Model file for the job. Use its own axes, mm. Face numbers are marked on the shaded views. A direction names the side the tool comes from. Give positions to 0.01 mm unless a question says otherwise; leave off trailing zeros. Order: outer loops, then holes, each group sorted by start corner. A loop starts at its lowest first (then second) coordinate and runs counter-clockwise, first axis right, second up. Notation, with made-up numbers: (53.25, 8) -> (79.25, 8) arc R22 ccw to (79.25, 40) -> close; hole circle Ø4 at (-27, -1.75). An arc over 180 degrees is marked (long way). Use CSV: the item, a comma, the result in double quotes. Start each with the question number.
1. Drop flat-ended pins along their axis: pin 1 (2 mm diameter, centred on x = 2.5, z = -27.5, fed in from +Y); pin 2 (2.5 mm diameter, centred on x = 1.5, y = -6.5, fed in from -Z); pin 3 (0.7 mm diameter, centred on x = 2, y = -9, fed in from -Z). Give the stop position or say it passes through.
2. Cut at D-D on z = -19. List the corners of the cut face in (x, y).
3. Cut at C-C on y = -13. List the corners of the cut face in (x, z), then the cut area to 3 significant figures.
4. Cut at A-A on x = 0.95. Give the number of separate pieces and of enclosed holes in the cut face, then the cut area to 3 significant figures.
5. Cut at B-B on z = -8. List the corners of the cut face in (x, y).
6. Wall check: line 1 (Z direction, x = 2.15, y = -14.5); line 2 (Y direction, x = 0.8, z = -1); line 3 (Y direction, x = 0.25, z = -3). Give the ranges that are in metal, low to high. Write a range as from..to.
7. 3-axis set-ups, long thin cutter, end or side, ignore diameter. For the marked faces 4, 5 and 6: which of +Z, -Z, +X, -X, +Y, -Y reach the whole face in a straight line?
8. Pull direction Y, two halves, no side cores. Call the marked faces 1, 2 and 3: released by +Y, released by -Y, zero draft, split by the parting line, or undercut.
```python
from build123d import *

# Parameters (mm, degrees)
F1_W     = 5
F1_H     = 5
F2_DEPTH = 5


with BuildPart() as f2:
    # F1 (on Right) → F2 (new body)
    with BuildSketch(Plane.YZ):
        with BuildLine():
            Line((-3.5, 0), (0, 0))
            Line((0, 0), (0, 8))
            ThreePointArc((0, 8), (-0.5857864376, 9.4142135624), (-2, 10))
            Line((-2, 10), (-20.8578643763, 10))
            ThreePointArc((-20.8578643763, 10), (-28.5115330236, 8.4775906502), (-35, 4.1421356237))
            Line((-35, 4.1421356237), (-66.0121933088, -26.8700576851))
            ThreePointArc((-66.0121933088, -26.8700576851), (-66.5979797464, -28.2842712475), (-66.0121933088, -29.6984848098))
            Line((-66.0121933088, -29.6984848098), (-61.7695526217, -33.941125497))
            ThreePointArc((-61.7695526217, -33.941125497), (-60.3553390593, -34.5269119346), (-58.941125497, -33.941125497))
            Line((-58.941125497, -33.941125497), (-25, 0))
            Line((-25, 0), (-21.5, 0))
            Line((-21.5, 0), (-16.5, 0))
            Line((-16.5, 0), (-14.1, 0))
            Line((-14.1, 0), (-14.1, 2.5))
            Line((-14.1, 2.5), (-15.25, 2.5))
            Line((-15.25, 2.5), (-15.25, 5))
            Line((-15.25, 5), (-12.5, 5))
            Line((-12.5, 5), (-9.75, 5))
            Line((-9.75, 5), (-9.75, 2.5))
            Line((-9.75, 2.5), (-10.9, 2.5))
            Line((-10.9, 2.5), (-10.9, 0))
            Line((-10.9, 0), (-8.5, 0))
            Line((-8.5, 0), (-3.5, 0))
        make_face()
        Polygon((-56.6225703117, -26.460690809), (-58.5317586209, -24.5515024998), (-54.9962247149, -21.0159685939), (-53.0870364057, -22.9251569031), align=None, mode=Mode.SUBTRACT)
        Polygon((-40.8540890912, -6.8738329701), (-37.3185551853, -3.3382990642), (-35.4093668761, -5.2474873734), (-38.944900782, -8.7830212793), align=None, mode=Mode.SUBTRACT)
        with Locations((-6, -2.5)):
            Rectangle(F1_W, F1_H)
        with Locations((-19, -2.5)):
            Rectangle(F1_W, F1_H)
    extrude(amount=F2_DEPTH)


solid = f2.part
```
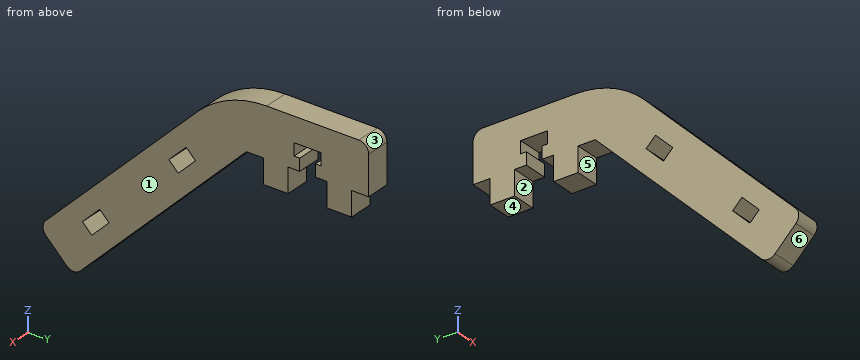
Verdict:
1,pin 1,"y = -51.5"
1,pin 2,"z = -5"
1,pin 3,"z = 0"
2,outline,"(0, -58.14) -> (5, -58.14) -> (5, -44) -> (0, -44) -> close"
3,outline,"(0, 5) -> (5, 5) -> (5, 10) -> (0, 10) -> close"
3,area,"25.0 mm^2"
4,separate pieces,"1"
4,enclosed holes,"2"
4,area,"781 mm^2"
5,outline,"(0, -47.14) -> (5, -47.14) -> (5, -39.73) -> (0, -39.73) -> close; (0, -38.16) -> (5, -38.16) -> (5, -33) -> (0, -33) -> close"
6,line 1,"0..2.5, 5..10"
6,line 2,"-40.14..-26, -21.5..-16.5, -8.5..-3.5"
6,line 3,"-42.14..-28, -21.5..-16.5, -8.5..-3.5"
7,face 4,"-Z, +X, -X, +Y"
7,face 5,"-Z, +X, -X"
7,face 6,"-Z, +X, -X, -Y"
8,face 1,"zero draft"
8,face 2,"undercut"
8,face 3,"released by +Y"
